Input: dimensioned drawing with shaded views. Units: mm. Origin: part minimum x, y, z. A direction names the side the tool comes from. Round coordinates to 2 decimals unless told otherwise and drop trailing zeros. Loops run counter-clockwise (first coordinate to the right, second up) from the corner with the lowest first, then second, coordinate; pieces in that order, holes last. Notation, with made-up numbers: M 36.5,-37.5 L 59.5,-37.5 A20 cw 59.5,-32.5 Z; hole C -23,-19.5 d8. An arc over 180 degrees is marked long. Answer as a JSON object with one key per item and string values.
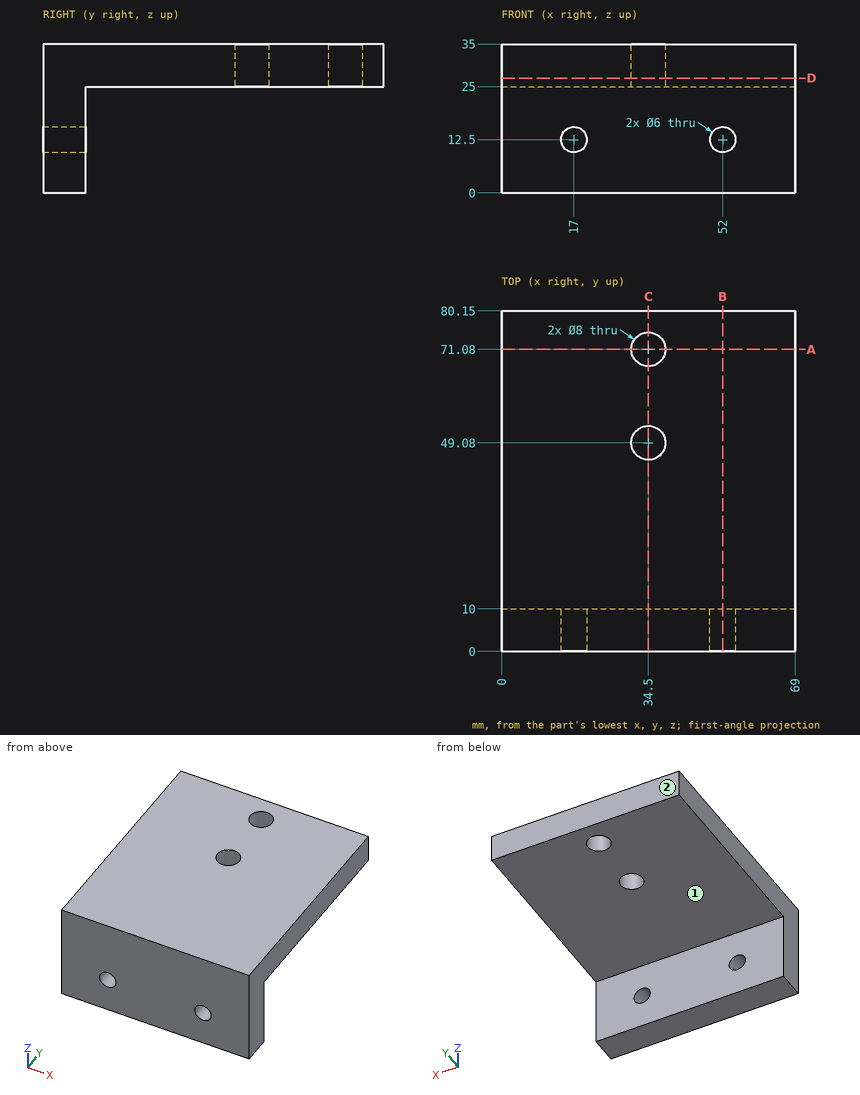
Item 1: Line query: probe 1 along Y at (x, z) = (34.5, 31); probe 2 along Z at (x, y) = (17, 5); probe 3 along Y at (x, z) = (39.5, 6). Output: solid intervals per line, ascending. Write a range as from..to.
Answer sheet:
{"probe 1": "y = 0..45.08, 53.08..67.08, 75.08..80.15", "probe 2": "z = 0..9.5, 15.5..35", "probe 3": "y = 0..10"}
Item 2: Section C-C on x = 34.5. Return the cut outline in (y, z).
Answer sheet:
{"outline": "M 0,0 L 10,0 L 10,25 L 45.08,25 L 45.08,35 L 0,35 Z; M 53.08,25 L 67.08,25 L 67.08,35 L 53.08,35 Z; M 75.08,25 L 80.15,25 L 80.15,35 L 75.08,35 Z"}
Item 3: Section D-D on z = 27. Return the cut outline in (x, y), then the cut area to 3 significant figures.
Answer sheet:
{"outline": "M 0,0 L 69,0 L 69,80.15 L 0,80.15 Z; hole C 34.5,49.08 d8; hole C 34.5,71.08 d8", "area": "5,430 mm²"}
Item 4: Section B-B on x = 52. Return the cut outline in (y, z), then the cut area to 4 significant figures.
Answer sheet:
{"outline": "M 0,0 L 10,0 L 10,9.5 L 0,9.5 Z; M 0,15.5 L 10,15.5 L 10,25 L 80.15,25 L 80.15,35 L 0,35 Z", "area": "991.5 mm²"}
Item 5: Contact query for flat-ended pins moving along their axis: pin 1 Ø20 at (x, z) = (46.5, 7.5) entering from +Y; pin 2 Ø8 at (x, y) = (24.5, 31) entering from -Z. Output: stop coordinate, or through.
Answer sheet:
{"pin 1": "stops at y = 10", "pin 2": "stops at z = 25"}
Item 6: Section A-A on y = 71.08. Return the cut outline in (x, z), then the cut area to 3 significant figures.
Answer sheet:
{"outline": "M 0,25 L 30.5,25 L 30.5,35 L 0,35 Z; M 38.5,25 L 69,25 L 69,35 L 38.5,35 Z", "area": "610 mm²"}
Item 7: Access query for the marked faces 1 and 2. Directions: +Z, -Z, +X, -X, +Y, -Y. A direction counts if a zero-diameter tool reaches every point of the face in a straight line with its end or side. Return the directions, or none.
Answer sheet:
{"face 1": "-Z, +X, -X, +Y", "face 2": "+Z, -Z, +X, -X, +Y"}
